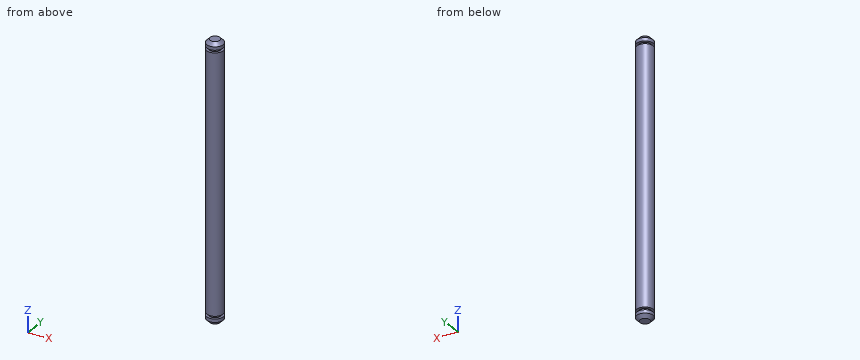
```python
from build123d import *

# Parameters (mm, degrees)
SKETCH_1_R      = 2.5
EXTRUDE_1_DEPTH = 41.5
SKETCH_2_W      = 0.75
SKETCH_2_H      = 0.8
CHAMFER_1_SIZE  = 1


with BuildPart() as part:
    # 草图1 → 凸台-拉伸1 (new, symmetric)
    with BuildSketch(Plane.XY):
        Circle(SKETCH_1_R)
    extrude(amount=EXTRUDE_1_DEPTH, both=True)

    # 草图2 → 切除-旋转1 (revolve, cut)
    with BuildSketch(Plane(origin=(0, 0, 0), x_dir=(1, 0, 0), z_dir=(0, 1, 0))):
        with Locations((2.125, 39.1)):
            Rectangle(SKETCH_2_W, SKETCH_2_H)
        with Locations((2.125, -39.1)):
            Rectangle(SKETCH_2_W, SKETCH_2_H)
    revolve(axis=Axis((0, 0, 49.423149105), (0, 0, -1)), mode=Mode.SUBTRACT)

    # 倒角1
    chamfer_1_edges = [part.edges().sort_by_distance(p)[0] for p in [
        (-2.5, 0, -41.5),
        (-2.5, 0, 41.5),
    ]]
    chamfer(chamfer_1_edges, length=CHAMFER_1_SIZE)


solid = part.part
```
The model under review builds one solid part; all positions refer to its coordinate system, in mm. Round coordinates to 2 decimals unless told otherwise and drop trailing zeros. Loops run counter-clockwise (first coordinate to the right, second up) from the corner with the lowest first, then second, coordinate; pieces in that order, holes last. Notation, with made-up numbers: (-17, -7.5) -> (42, -7.5) arc R23 ccw to (42, 9.5) -> close; hole circle Ø5 at (-38.75, 43). An arc over 180 degrees is marked (long way). Answer as a JSON object with one key per item and string values. Group by question number.
1) For line 1 (Z direction, x = 1.25, y = -1.4); line 2 (Z direction, x = -1.8, y = -1.05); line 3 (X direction, y = -1.8, z = -19.5), list the stretches that pass through material, from the lowest coordinate up. Write a range as [from, to].
2) For pin 1 Ø1.5 at (y, z) = (-2, -16) entering from -X, flat-tipped, find the tip position at first contact; note if it passes through.
3) We need section A-A on z = 6.5. Write out the cut boundary in (x, y).
Result set:
{
 "1": {"line 1": "[-41.12, -39.5], [-38.7, 38.7], [39.5, 41.12]", "line 2": "[-40.92, -39.5], [-38.7, 38.7], [39.5, 40.92]", "line 3": "[-1.73, 1.73]"},
 "2": {"pin 1": "x = -2.17"},
 "3": {"outline": "circle Ø5 at (0, 0)"}
}
